```python
from build123d import *

# Parameters (mm, degrees)
SKETCH19_R         = 4
CUT_EXTRUDE3_DEPTH = 25.4


with BuildPart() as part:
    # Sketch1 → Revolve1 (revolve)
    with BuildSketch(Plane.XY):
        with BuildLine():
            Line((0, 0), (0, 11.938))
            Line((0, 11.938), (24.765, 11.938))
            ThreePointArc((24.765, 11.938), (26.561051224, 12.681948776), (27.305, 14.478))
            Line((27.305, 14.478), (27.305, 22.933028409))
            Line((27.305, 22.933028409), (28.104406531, 23.876))
            Line((28.104406531, 23.876), (57.15, 23.876))
            Line((57.15, 23.876), (57.15, 49.2125))
            Line((57.15, 49.2125), (759.206, 49.2125))
            Line((759.206, 49.2125), (759.206, 0))
            Line((759.206, 0), (0, 0))
        make_face()
    revolve(axis=Axis((759.206, 0, 0), (-1, 0, 0)))

    # Sketch16 → Cut-Revolve1 (revolve, cut)
    with BuildSketch(Plane(origin=(0, 0, 0), x_dir=(1, 0, 0), z_dir=(0, 1, 0))):
        Polygon((0, 0), (0, 8.35025), (1.905, 6.556375), (1.905, 0), align=None)
    revolve(axis=Axis((1.905, 0, 0), (-1, 0, 0)), mode=Mode.SUBTRACT)

    # Sketch19 → Cut-Extrude3 (cut)
    with BuildSketch(Plane.ZY.offset(-1.905)):
        Circle(SKETCH19_R)
    extrude(amount=-CUT_EXTRUDE3_DEPTH, mode=Mode.SUBTRACT)

    # Sketch32 → Cut-Revolve6 (revolve, cut)
    with BuildSketch(Plane(origin=(0, 0, 0), x_dir=(1, 0, 0), z_dir=(0, 1, 0)), mode=Mode.PRIVATE) as cut_revolve6_sk:
        Polygon((27.305, 0), (28.575, 0), (27.305, 6.351059428), align=None)
    revolve(cut_revolve6_sk.sketch.rotate(Axis((27.305, 0, 0), (1, 0, 0)), 180), axis=Axis((27.305, 0, 0), (1, 0, 0)), mode=Mode.SUBTRACT)


solid = part.part
```
The listing builds one solid part. Answer for the finished solid, in the listing's coordinates (mm). A direction names the side the tool comes from. Give positions to 0.01 mm unless a question says otherwise; leave off trailing zeros. Loops run counter-clockwise (first coordinate to the right, second up) from the corner with the lowest first, then second, coordinate; pieces in that order, holes last. Notation, with made-up numbers: (28.5, 23.5) - (78.5, 23.5) arc R17 cw to (78.5, 27.5) - close; hole circle Ø2 at (30.5, 20). An arc over 180 degrees is marked (long way). Return JSON: item names as keys, results as strings. Group by question number.
1. Straight lines are drawn through the part: line 1 (Y direction, x = 16.75, z = 0); line 2 (X direction, y = -32, z = 7); line 3 (X direction, y = 22, z = 7). For each, find the intervals that lie inside material, in ascending order. Write a range as [from, to].
2. Find section A-A (x = 220). Write down the section's boundary in (y, z) (1 decimal).
3. Which of the six approach directions +Z, -Z, +X, -X, +Y, -Y give full straight-line access (tool end or side, diameter ignored) to faces 4 (the flat face through (27.305, 0, 15)), 5 (the cylindrical face through (413.09, 46.94, -14.78)), 6 (the conical face through (28.496, 0.352, 0.183))?
4. Find section B-B (y = -40.5). Write down the section's boundary in (x, z).
5. Given pin 1 Ø3 at (x, y) = (624.5, -38) entering from -Z; pin 2 Ø10.5 at (y, z) = (2, 0) entering from -X; pin 3 Ø5 at (x, z) = (168.5, -27) entering from -Y, each flat-ended and moving along its own axis, determine where each tip first touches the part or whether it passes through.
6. Determine the mould class of faces 1 (the flat face through (57.15, 12, 21)), 2 (the flat face through (1.905, 3, 3)), 3 (the cylindrical face through (42.831, -5.176, 23.308)) for opening direction Z: pulls with the +Z half, pulls with the -Z half, needs draft (parallel to the pull), parting line crosses it, or undercut.
7. Find section C-C (z = 38.5). Write down the section's boundary in (x, y).
Verdict:
{
 "1": {"line 1": "y = [-11.94, -4], [4, 11.94]", "line 2": "x = [57.15, 759.21]", "line 3": "x = [27.44, 759.21]"},
 "2": {"outline": "circle Ø98.4 at (0, 0)"},
 "3": {"face 4": "-X", "face 5": "+X, -X", "face 6": "none"},
 "4": {"outline": "(57.15, -27.96) - (759.21, -27.96) - (759.21, 27.96) - (57.15, 27.96) - close"},
 "5": {"pin 1": "stops at z = -33.01", "pin 2": "stops at x = 1.17", "pin 3": "stops at y = -42.68"},
 "6": {"face 1": "needs draft", "face 2": "undercut", "face 3": "parting line crosses it"},
 "7": {"outline": "(57.15, -30.65) - (759.21, -30.65) - (759.21, 30.65) - (57.15, 30.65) - close"}
}
